Can you work these out from the model? Positions are in its coordinate system, mm. Give positions to 0.01 mm unless a question says otherwise; leave off trailing zeros.
Autodesk Inventor part; units mm, degrees
ref_plane "YZ Plane" through (0, 0, 0) normal (1, 0, 0) x (0, 1, 0)
ref_plane "XZ Plane" through (0, 0, 0) normal (0, 1, 0) x (-1, 0, 0)
ref_plane "XY Plane" through (0, 0, 0) normal (0, 0, 1) x (1, 0, 0)
sketch "Sketch1" plane through (0, 0, 0) normal (0, 0, 1) x (1, 0, 0)
  line L0 (-125, 12.5) -> (125, 12.5)
  line L1 (125, 12.5) -> (125, -12.5)
  line L2 (125, -12.5) -> (-125, -12.5)
  line L3 (-125, -12.5) -> (-125, 12.5)
  line L4 (-125, 12.5) -> (125, -12.5) construction
  line L5 (125, 12.5) -> (-125, -12.5) construction
  line L6 (100, -5) -> (-100, -5)
  line L7 (-100, -5) -> (-100, 5)
  line L8 (-100, 5) -> (100, 5)
  line L9 (100, 5) -> (100, -5)
  line L10 (100, -5) -> (-100, 5) construction
  line L11 (-100, -5) -> (100, 5) construction
  line L12 (-120, 12.5) -> (-120, 15.7)
  line L13 (-120, 15.7) -> (-105, 15.7)
  line L14 (-105, 15.7) -> (-105, 12.5)
  line L15 (-7.5, 12.5) -> (-7.5, 15.7)
  line L16 (-7.5, 15.7) -> (7.5, 15.7)
  line L17 (7.5, 15.7) -> (7.5, 12.5)
  line L18 (0, 0) -> (0, 12.5) construction
  line L19 (0, 0) -> (31.571, 0) construction
  line L20 (120, 12.5) -> (120, 15.7)
  line L21 (120, 15.7) -> (105, 15.7)
  line L22 (105, 15.7) -> (105, 12.5)
  line L23 (-120, -12.5) -> (-120, -15.7)
  line L24 (-120, -15.7) -> (-105, -15.7)
  line L25 (-105, -15.7) -> (-105, -12.5)
  line L26 (-7.5, -12.5) -> (-7.5, -15.7)
  line L27 (-7.5, -15.7) -> (7.5, -15.7)
  line L28 (7.5, -15.7) -> (7.5, -12.5)
  line L29 (120, -12.5) -> (120, -15.7)
  line L30 (120, -15.7) -> (105, -15.7)
  line L31 (105, -15.7) -> (105, -12.5)
  circle A0 centre (-116, 0) radius 2
  circle A1 centre (-116, 0) radius 2
  circle A2 centre (116, 0) radius 2
  line L32 (-12.5, 5) -> (12.5, 5)
  line L33 (12.5, 5) -> (12.5, -5)
  line L34 (12.5, -5) -> (-12.5, -5)
  line L35 (-12.5, -5) -> (-12.5, 5)
  line L36 (-12.5, 5) -> (12.5, -5) construction
  line L37 (12.5, 5) -> (-12.5, -5) construction
  dimension "d0" = 250
  dimension "d1" = 25
  dimension "d6" = 200
  dimension "d7" = 10
  dimension "d10" = 3.2
  dimension "d11" = 15
  dimension "d12" = 5
  dimension "d13" = 3.2
  dimension "d14" = 15
  dimension "d15" = 7.5
  dimension "d18" = 25
  dimension "d19" = 10
extrude "Extrusion4" add sketch "Sketch1" along normal blind 3.2 contours L0 L1 L2 L3 | L12 L13 L14 L0 | L2 L25 L24 L23 | L15 L16 L17 L0 | L2 L28 L27 L26 | L22 L21 L20 L0 | L2 L29 L30 L31 | L6 L35 L8 L33
properties part number "Base_Carril"
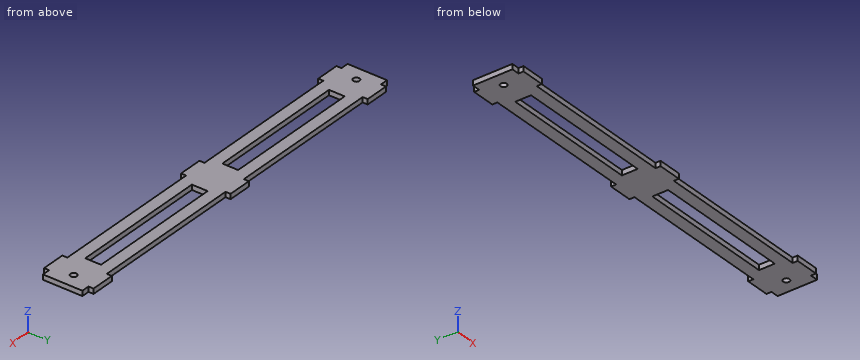
(1) Will these pins go through, and if not, where does the flat tip stop? P1, Ø1, axis at y = -14.5, z = 1, coming from the -X side; P2, Ø3, axis at x = -52.5, y = 4, coming from the -Z side; P3, Ø1.6, axis at x = -123, z = 2, coming from the +Y side; P4, Ø1.6, axis at y = -15, z = 1.5, coming from the +X side.
Returned:
P1: stops at x = -120
P2: stops at z = 0
P3: stops at y = 12.5
P4: stops at x = 120
(2) Please list where these lines run through material, in increasing order: probe 1 along X at (y, z) = (4, 2.3); probe 2 along Y at (x, z) = (-116, 1.2); probe 3 along Y at (x, z) = (-63.5, 1).
Returned:
probe 1: x = -125 to -100, -12.5 to 12.5, 100 to 125
probe 2: y = -15.7 to -2, 2 to 15.7
probe 3: y = -12.5 to -5, 5 to 12.5
(3) Suppose I cut it at A-A on z = 1.8. Give the number of separate pieces and of enclosed holes in the cut face, plus the area to 3 significant figures.
Returned:
separate pieces: 1
enclosed holes: 4
area: 4,760 mm2
